Check sheet for the modelled part. Datum: model origin and axes. Units: mm. A direction names the side the tool comes from. Round coordinates to 2 decimals unless told otherwise and drop trailing zeros. Write each loop counter-clockwise with the first axis right and the second up, starting at its lowest first coordinate (ties: lowest second). Pieces come first, ordered by that corner, then holes. Notation, with made-up numbers: (11.25, -10.5) -> (20.25, -10.5) arc R13 cw to (20.25, -1.5) -> close; hole circle Ø10 at (69, -7). An arc over 180 degrees is marked (long way). One line per item, written item: value.
from build123d import *

# Parameters (mm, degrees)
F0_W      = 127
F0_H      = 120.65
F1_DEPTH  = 139.7
F2_W      = 76.2
F2_H      = 57.15
F3_DEPTH  = 76.2
F5_DEPTH  = 127.001
F6_W      = 50.8
F6_H      = 57.15
F7_DEPTH  = 25.4
F9_R      = 12.7
F10_DEPTH = 215.901
F11_R     = 12.7
F12_DEPTH = 127.001


with BuildPart() as f1:
    # F0 (on Right) → F1 (new body)
    with BuildSketch(Plane.YZ):
        Rectangle(F0_W, F0_H)
    extrude(amount=F1_DEPTH)

    # F2 (on face) → F3 (join)
    with BuildSketch(Plane(origin=(0, 0, 0), x_dir=(0, -1, 0), z_dir=(-1, 0, 0))):
        with Locations((25.4, 31.75)):
            Rectangle(F2_W, F2_H)
    extrude(amount=F3_DEPTH)

    # F4 (on face) → F5 (cut, through all)
    with BuildSketch(Plane.XZ.offset(63.5)):
        with BuildLine():
            ThreePointArc((19.05, 60.325), (104.362433, 24.987433), (139.7, -60.325))
            Line((139.7, -60.325), (139.7, 60.325))
            Line((139.7, 60.325), (19.05, 60.325))
        make_face()
    extrude(amount=-F5_DEPTH, mode=Mode.SUBTRACT)

    # F6 (on face) → F7 (join)
    with BuildSketch(Plane(origin=(0, 0, 0), x_dir=(0, -1, 0), z_dir=(-1, 0, 0))):
        with Locations((-38.1, 31.75)):
            Rectangle(F6_W, F6_H)
    extrude(amount=F7_DEPTH)

    # F9 (on face) → F10 (cut, through all)
    with BuildSketch(Plane(origin=(-76.2, 0, 0), x_dir=(0, -1, 0), z_dir=(-1, 0, 0))):
        with Locations((25.187448, 28.472066)):
            Circle(F9_R)
    extrude(amount=-F10_DEPTH, mode=Mode.SUBTRACT)

    # F11 (on face) → F12 (cut, through all)
    with BuildSketch(Plane.XZ.offset(63.5)):
        with Locations((76.003939, -15.616879)):
            Circle(F11_R)
    extrude(amount=-F12_DEPTH, mode=Mode.SUBTRACT)


solid = f1.part
Item 1: Sectioned sample at A-A (x = 68). Enter the section's corners in (y, z) (1 decimal), then the cut area to 3 significant figures.
Result set:
outline: (-63.5, -60.3) -> (63.5, -60.3) -> (63.5, -25.5) -> (-63.5, -25.5) -> close; (-63.5, -5.8) -> (63.5, -5.8) -> (63.5, 49.9) -> (-63.5, 49.9) -> close; hole circle Ø25.4 at (-25.2, 28.5)
area: 11,000 mm^2
Item 2: Sectioned sample at B-B (y = 28). Enter the section's corners in (x, z) (3 decimals).
Result set:
outline: (-25.4, 3.175) -> (0, 3.175) -> (0, -60.325) -> (139.7, -60.325) arc R120.65 ccw to (19.05, 60.325) -> (-25.4, 60.325) -> close; hole circle Ø25.4 at (76.004, -15.617)
Item 3: Release check for a two-part mould opening along Z. For faces 1 (the flat face through (-25.4, 38, 32)), 2 (the cylindrical face through (16.918, -31.048, 17.205)), 3 (the cylindrical face through (65.926, -0.889, -23.345)), 4 (the flat face through (-29, -13, 3.175)) record: pulls with the +Z half, pulls with the -Z half, needs draft (parallel to the pull), parting line crosses it, or undercut.
Result set:
face 1: needs draft
face 2: undercut
face 3: undercut
face 4: pulls with the -Z half
Item 4: Material ranges on line 1 along Z through (x, y) = (54, -30) (3 decimals); line 2 along Z through (x, y) = (-9, -35.5) (3 decimals); line 3 along X through (y, z) = (43.5, -16), recorded low to high.
Result set:
line 1: -60.325 to 16.719, 40.225 to 55.152
line 2: 3.175 to 21.06, 35.884 to 60.325
line 3: 0 to 63.31, 88.7 to 131.26
Item 5: Tool access check on faces 5 (the flat face through (-50, 12.7, 31)), 6 (the flat face through (0, -1, -28)), 7 (the flat face through (-76.2, -16, 39)). Record the directions out of +Z, -Z, +X, -X, +Y, -Y that give a thin tool (end or side, any length) a straight path to the whole face; none if there is none.
Result set:
face 5: +Z, -Z, -X, +Y
face 6: -Z, -X, +Y, -Y
face 7: +Z, -Z, -X, +Y, -Y
Item 6: Sectioned sample at D-D (z = -35.5). Enter the section's corners in (x, y), then the cut area to 3 significant figures.
Result set:
outline: (0, -63.5) -> (137.12, -63.5) -> (137.12, 63.5) -> (0, 63.5) -> close
area: 17,400 mm^2
Item 7: Sectioned sample at C-C (x = 11). Enter the section's corners in (y, z) (3 decimals).
Result set:
outline: (-63.5, -60.325) -> (63.5, -60.325) -> (63.5, 60.325) -> (-63.5, 60.325) -> close; hole circle Ø25.4 at (-25.187, 28.472)
Item 8: Depth check by flat-ended pin: pin 1 (1 mm diameter, centred on y = 42.5, z = 6, fed in from +X); pin 2 (3 mm diameter, centred on x = -41.5, y = -13, fed in from -Z) (3 decimals); pin 3 (6 mm diameter, centred on y = -39, z = -2, fed in from +X). Enter the tip coordinate at first touch or a pass-through.
Result set:
pin 1: x = 120.16
pin 2: z = 3.175
pin 3: x = 126.27
